Geometry: final body of the model. Coordinates: model frame, mm. Face numbers are marked on the shaded views. A direction names the side the tool comes from. Give positions to 0.01 mm unless a question says otherwise; leave off trailing zeros. Loops run counter-clockwise (first coordinate to the right, second up) from the corner with the lowest first, then second, coordinate; pieces in that order, holes last. Notation, with made-up numbers: M 69.5,-0.75 L 125.5,-0.75 A16 cw 125.5,10.25 Z; hole C 65,-11.5 d3. An arc over 180 degrees is marked long. Put each result on its own line as item: value.
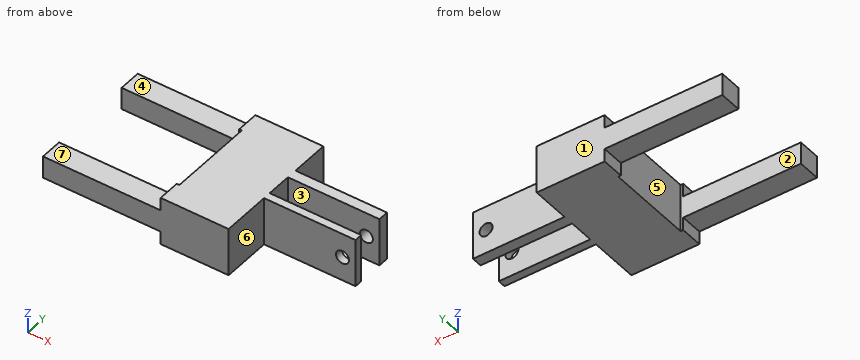
```python
from build123d import *

# Parameters (mm, degrees)
SKETCH_1_W          = 92
SKETCH_1_H          = 17
SKETCH_1_W_2        = 70
SKETCH_1_H_2        = 8
SKETCH_1_H_3        = 6
EXTRUDE_1_DEPTH     = 37
SKETCH_2_R          = 5
CUT_EXTRUDE_1_DEPTH = 142.57603411
SKETCH_3_W          = 10
SKETCH_3_H          = 17
CUT_EXTRUDE_2_DEPTH = 90


with BuildPart() as part:
    # 草图1 → 凸台-拉伸1 (new body)
    with BuildSketch(Plane.XY):
        with Locations((-71, 41.5)):
            Rectangle(SKETCH_1_W, SKETCH_1_H)
        with Locations((-71, -41.5)):
            Rectangle(SKETCH_1_W, SKETCH_1_H)
        with Locations((60, 16.610009448)):
            Rectangle(SKETCH_1_W_2, SKETCH_1_H_2)
        with Locations((60, -9.610009448)):
            Rectangle(SKETCH_1_W_2, SKETCH_1_H_3)
        Polygon((25, 50), (-25, 50), (-25, 33), (-25, -33), (-25, -50), (25, -50), (25, -12.610009448), (25, -6.610009448), (25, 12.610009448), (25, 20.610009448), align=None)
    extrude(amount=EXTRUDE_1_DEPTH)

    # 草图2 → 切除-拉伸1 (cut, through all)
    with BuildSketch(Plane(origin=(0, 20.610009448, 0), x_dir=(1, 0, 0), z_dir=(0, 1, 0))):
        with Locations(Location((85, -18.5, 0), (0, 0, 270))):
            Circle(SKETCH_2_R)
    extrude(amount=-CUT_EXTRUDE_1_DEPTH, mode=Mode.SUBTRACT)

    # 草图3 → 切除-拉伸2 (cut)
    with BuildSketch(Plane.ZY.offset(117)):
        with Locations((5, -41.5)):
            Rectangle(SKETCH_3_W, SKETCH_3_H)
        with Locations((32, -41.5)):
            Rectangle(SKETCH_3_W, SKETCH_3_H)
        with Locations((32, 41.5)):
            Rectangle(SKETCH_3_W, SKETCH_3_H)
        with Locations((5, 41.5)):
            Rectangle(SKETCH_3_W, SKETCH_3_H)
    extrude(amount=-CUT_EXTRUDE_2_DEPTH, mode=Mode.SUBTRACT)


solid = part.part
```
Item 1: Section D-D on y = -36. Output: boundary loops of the cut face in (x, z).
Output values:
outline: M -117,10 L -27,10 L -27,0 L 25,0 L 25,37 L -27,37 L -27,27 L -117,27 Z
Item 2: Section B-B on x = -31.5. Output: boundary loops of the cut face in (y, z), then the cut area to 3 significant figures.
Output values:
outline: M -50,10 L -33,10 L -33,27 L -50,27 Z; M 33,10 L 50,10 L 50,27 L 33,27 Z
area: 578 mm²
Item 3: Line query: probe 1 along Y at (x, z) = (64.5, 13); probe 2 along X at (y, z) = (18, 18.5); probe 3 along Y at (x, z) = (-48, 13). Output: solid intervals per line, ascending. Write a range as [from, to].
Output values:
probe 1: [-12.61, -6.61], [12.61, 20.61]
probe 2: [-25, 80], [90, 95]
probe 3: [-50, -33], [33, 50]
Item 4: Set-up query: the marked faces 5, 6 and 7. Return all of +Z, -Z, +X, -X, +Y, -Y with unobstructed straight access to the full face (end or side cutting, diameter ignored); none if empty.
Output values:
face 5: +Z, -Z, -X
face 6: +Z, -Z, +X, -Y
face 7: +Z, -X, +Y, -Y
Item 5: Section C-C on x = 85. Output: boundary loops of the cut face in (y, z).
Output values:
outline: M -12.61,0 L -6.61,0 L -6.61,13.5 L -12.61,13.5 Z; M -12.61,23.5 L -6.61,23.5 L -6.61,37 L -12.61,37 Z; M 12.61,0 L 20.61,0 L 20.61,13.5 L 12.61,13.5 Z; M 12.61,23.5 L 20.61,23.5 L 20.61,37 L 12.61,37 Z
Item 6: Mould query, pull axis Y, two halves, no side actions, for the marked faces 1, 2, 3 and 4. Classes: pulls with the +Y half, pulls with the -Y half, needs draft (parallel to the pull), parting line crosses it, or undercut.
Output values:
face 1: pulls with the +Y half
face 2: undercut
face 3: undercut
face 4: needs draft
Item 7: Section A-A on z = 21.5. Output: boundary loops of the cut face in (x, y).
Output values:
outline: M -117,-50 L 25,-50 L 25,-12.61 L 81,-12.61 L 81,-6.61 L 25,-6.61 L 25,12.61 L 81,12.61 L 81,20.61 L 25,20.61 L 25,50 L -117,50 L -117,33 L -25,33 L -25,-33 L -117,-33 Z; M 89,-12.61 L 95,-12.61 L 95,-6.61 L 89,-6.61 Z; M 89,12.61 L 95,12.61 L 95,20.61 L 89,20.61 Z
Item 8: Pin query (flat end, axial travel): pin 1 Ø5 at (x, y) = (-87.5, 45) entering from +Z; pin 2 Ø10 at (x, y) = (29.5, 21) entering from -Z; pin 3 Ø3 at (y, z) = (-43.5, 32.5) entering from -X; pin 4 Ø6 at (y, z) = (5, 11) entering from +X. Return the tip coordinate at first contact, or that it passes through.
Output values:
pin 1: z = 27
pin 2: z = 0
pin 3: x = -27
pin 4: x = 25
